from build123d import *

# Parameters (mm, degrees)
SKETCH_R        = 2.55
PAD_DEPTH       = 10
SKETCH001_R     = 1
POCKET_DEPTH    = 6
SKETCH002_W     = 8.6
SKETCH002_H     = 2
SKETCH002_W_2   = 7.1
POCKET001_DEPTH = 32.001
POCKET002_DEPTH = 4
SKETCH004_R     = 6.2
POCKET003_DEPTH = 3


with BuildPart() as part:
    # Sketch → Pad (new body)
    with BuildSketch(Plane.XY):
        Polygon((0, 21.5), (0, 0), (32, 0), (32, 20), (17, 20), (17, 21.5), align=None)
        with Locations((24.5, 10)):
            Circle(SKETCH_R, mode=Mode.SUBTRACT)
    extrude(amount=PAD_DEPTH)

    # Sketch001 (on Face9 of Pad) → Pocket (cut)
    with BuildSketch(Plane.XY.offset(10)):
        with BuildLine():
            Line((2, 21.5), (15, 21.5))
            Line((15, 21.5), (15, 15))
            Line((13.110147, 15), (15, 15))
            ThreePointArc((10.389853, 15), (11.75, 14.5), (13.110147, 15))
            Line((8.5, 15), (10.389853, 15))
            Line((8.5, 15), (6.610147, 15))
            ThreePointArc((3.889853, 15), (5.25, 14.5), (6.610147, 15))
            Line((2, 15), (3.889853, 15))
            Line((2, 15), (2, 21.5))
        make_face()
        with Locations((5.25, 16.6)):
            Circle(SKETCH001_R, mode=Mode.SUBTRACT)
        with Locations((11.75, 16.6)):
            Circle(SKETCH001_R, mode=Mode.SUBTRACT)
    extrude(amount=-POCKET_DEPTH, mode=Mode.SUBTRACT)

    # Sketch002 (on Face1 of Pocket) → Pocket001 (cut, through all)
    with BuildSketch(Plane(origin=(0, 0, 0), x_dir=(0, -1, 0), z_dir=(-1, 0, 0))):
        with Locations((-17.2, 1)):
            Rectangle(SKETCH002_W, SKETCH002_H)
        with Locations((-3.55, 1)):
            Rectangle(SKETCH002_W_2, SKETCH002_H)
    extrude(amount=-POCKET001_DEPTH, mode=Mode.SUBTRACT)

    # Sketch003 (on Face8 of Pocket001) → Pocket002 (cut)
    with BuildSketch(Plane.XY.offset(10)):
        with BuildLine():
            Line((7.75, 15), (7.75, 9.5))
            Line((7.75, 9.5), (7.99, 9.26))
            Line((7.99, 3.6), (7.99, 9.26))
            Line((5.01, 3.6), (7.99, 3.6))
            ThreePointArc((4.01, 4.6), (4.302893, 3.892893), (5.01, 3.6))
            Line((4.01, 9.26), (4.01, 4.6))
            Line((4.25, 9.5), (4.01, 9.26))
            Line((4.25, 15), (4.25, 9.5))
            Line((2.75, 15), (4.25, 15))
            Line((2.75, 15), (2.75, 9.5))
            Line((2.75, 9.5), (2.99, 9.26))
            Line((2.99, 9.26), (2.99, 3.8))
            ThreePointArc((2.99, 3.8), (3.517208, 2.527208), (4.79, 2))
            Line((4.79, 2), (32, 2))
            Line((32, 2), (32, 3.6))
            Line((32, 3.6), (15.01, 3.6))
            ThreePointArc((14.01, 4.6), (14.302893, 3.892893), (15.01, 3.6))
            Line((14.01, 4.6), (14.01, 9.26))
            Line((14.01, 9.26), (14.25, 9.5))
            Line((14.25, 9.5), (14.25, 15))
            Line((14.25, 15), (12.75, 15))
            Line((12.75, 15), (12.75, 9.5))
            Line((12.75, 9.5), (12.99, 9.26))
            Line((12.99, 9.26), (12.99, 3.6))
            Line((12.99, 3.6), (10.01, 3.6))
            ThreePointArc((9.01, 4.6), (9.302893, 3.892893), (10.01, 3.6))
            Line((9.01, 4.6), (9.01, 9.26))
            Line((9.01, 9.26), (9.25, 9.5))
            Line((9.25, 9.5), (9.25, 15))
            Line((9.25, 15), (7.75, 15))
        make_face()
    extrude(amount=-POCKET002_DEPTH, mode=Mode.SUBTRACT)

    # Sketch004 (on Face23 of Pocket002) → Pocket003 (cut)
    with BuildSketch(Plane.XY.offset(10)):
        with Locations((24.5, 10)):
            Circle(SKETCH004_R)
    extrude(amount=-POCKET003_DEPTH, mode=Mode.SUBTRACT)


solid = part.part
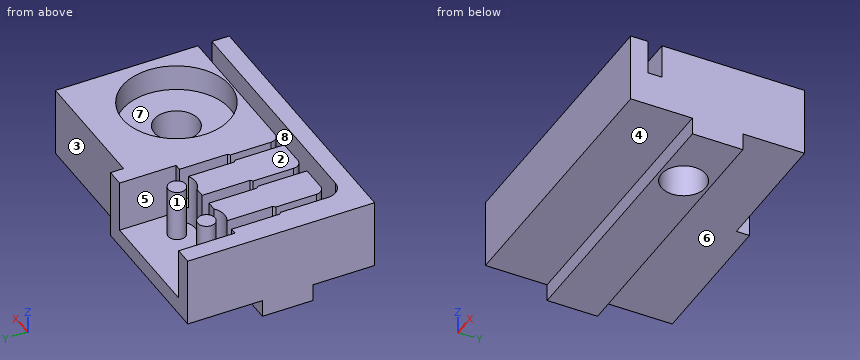
Here's how the part is built. I have some questions about the finished solid (model axes, mm). Face numbers are marked on the shaded views. A direction names the side the tool comes from. Coordinates: 2 decimals unless noted, no trailing zeros. Write each loop counter-clockwise with the first axis right and the second up, starting at its lowest first coordinate (ties: lowest second). Pieces come first, ordered by that corner, then holes.
1) If we section it at B-B (z = 1): List the corners of the cut face in (x, y) for me, plus the area to 3 significant figures.
Filled in:
outline: (0, 7.1) - (32, 7.1) - (32, 12.9) - (0, 12.9) - close; hole circle Ø5.1 at (24.5, 10)
area: 165 mm2
2) If we section it at C-C (x = 26): List the corners of the cut face in (y, z) for me, plus the area to 3 significant figures.
Filled in:
outline: (0, 2) - (7.1, 2) - (7.1, 0) - (7.94, 0) - (7.94, 7) - (3.98, 7) - (3.98, 10) - (3.6, 10) - (3.6, 6) - (2, 6) - (2, 10) - (0, 10) - close; (12.06, 0) - (12.9, 0) - (12.9, 2) - (20, 2) - (20, 10) - (16.02, 10) - (16.02, 7) - (12.06, 7) - close
area: 100 mm2
3) Thinking about a two-plate mould opening in Y: for the marked faces 1, 2 and 3, which applies, +Y half, -Y half, draft (parallel to the pull), parting line (faces both ways), or undercut?
Filled in:
face 1: undercut
face 2: draft
face 3: +Y half
4) Which directions (+Z, -Z, +X, -X, +Y, -Y) give clear straight access to the entire face, cutting with the end or side of a thin tool? Please do the marked faces 4, 5, 6, 7 and 8.
Filled in:
face 4: -Z, +X, -X, -Y
face 5: +Z, +Y
face 6: -Z, +X, -X, +Y
face 7: +Z
face 8: +Z, +X
5) If I drill on line 1 (X direction, y = 5.25, z = 6.75); line 2 (X direction, y = 16.5, z = 4.75); line 3 (X direction, y = 10, z = 3), over which ranges is the centre line in solid material (lowest first)?
Filled in:
line 1: x = 0 to 2.99, 4.01 to 7.99, 9.01 to 12.99, 14.01 to 32
line 2: x = 0 to 2, 4.26 to 6.24, 10.76 to 12.74, 15 to 32
line 3: x = 0 to 21.95, 27.05 to 32
6) If we section it at A-A (y = 10): List the corners of the cut face in (x, z) for me.
Filled in:
outline: (0, 0) - (21.95, 0) - (21.95, 7) - (18.3, 7) - (18.3, 10) - (14.25, 10) - (14.25, 6) - (12.75, 6) - (12.75, 10) - (9.25, 10) - (9.25, 6) - (7.75, 6) - (7.75, 10) - (4.25, 10) - (4.25, 6) - (2.75, 6) - (2.75, 10) - (0, 10) - close; (27.05, 0) - (32, 0) - (32, 10) - (30.7, 10) - (30.7, 7) - (27.05, 7) - close
7) I'm going to push flat-ended pins straight in: pin 1 (3.5 mm diameter, centred on x = 9, y = 19, fed in from +Z); pin 2 (0.9 mm diameter, centred on x = 13.5, z = 7.5, fed in from +Y); pin 3 (0.6 mm diameter, centred on x = 2.5, z = 8.5, fed in from +Y). Where does each tip first touch, or does it pass through?
Filled in:
pin 1: stops at z = 4
pin 2: stops at y = 2
pin 3: stops at y = 15
8) If we section it at D-D (z = 8.75): Count the separate pieces of the cut face and the enclosed holes in it, plus the area to 3 significant figures.
Filled in:
separate pieces: 6
enclosed holes: 1
area: 375 mm2
